from build123d import *

# Parameters (mm, degrees)
SKETCH1_W           = 16
SKETCH1_H           = 25
SKETCH1_W_2         = 11
SKETCH1_H_2         = 20
BOSS_EXTRUDE2_DEPTH = 2.5
SKETCH1_4_W         = 2.5
SKETCH1_4_H         = 2.5
BOSS_EXTRUDE3_DEPTH = 40
BOSS_EXTRUDE4_START = 40
SKETCH1_5_W         = 2.5
SKETCH1_5_H         = 20
SKETCH1_5_H_2       = 2.5
SKETCH1_5_W_2       = 11
BOSS_EXTRUDE4_DEPTH = 2.5


with BuildPart() as part:
    # Sketch1 → Boss-Extrude2 (new body)
    with BuildSketch(Plane(origin=(0, 0, 0), x_dir=(1, 0, 0), z_dir=(0, 1, 0))):
        with Locations((-8, 12.5)):
            Rectangle(SKETCH1_W, SKETCH1_H)
        with Locations((-8, 12.5)):
            Rectangle(SKETCH1_W_2, SKETCH1_H_2, mode=Mode.SUBTRACT)
    extrude(amount=BOSS_EXTRUDE2_DEPTH)

    # Sketch1_4 → Boss-Extrude3 (add)
    with BuildSketch(Plane(origin=(0, 0, 0), x_dir=(1, 0, 0), z_dir=(0, 1, 0))):
        with Locations((-14.75, 23.75)):
            Rectangle(SKETCH1_4_W, SKETCH1_4_H)
        with Locations((-14.75, 1.25)):
            Rectangle(SKETCH1_4_W, SKETCH1_4_H)
        with Locations((-1.25, 1.25)):
            Rectangle(SKETCH1_4_W, SKETCH1_4_H)
        with Locations((-1.25, 23.75)):
            Rectangle(SKETCH1_4_W, SKETCH1_4_H)
    extrude(amount=BOSS_EXTRUDE3_DEPTH)

    # Sketch1_5 → Boss-Extrude4 (add)
    with BuildSketch(Plane(origin=(0, 0, 0), x_dir=(1, 0, 0), z_dir=(0, 1, 0)).offset(BOSS_EXTRUDE4_START)):
        with Locations((-1.25, 12.5)):
            Rectangle(SKETCH1_5_W, SKETCH1_5_H)
        with Locations((-1.25, 1.25)):
            Rectangle(SKETCH1_5_W, SKETCH1_5_H_2)
        with Locations((-8, 1.25)):
            Rectangle(SKETCH1_5_W_2, SKETCH1_5_H_2)
        with Locations((-14.75, 1.25)):
            Rectangle(SKETCH1_5_W, SKETCH1_5_H_2)
        with Locations((-14.75, 12.5)):
            Rectangle(SKETCH1_5_W, SKETCH1_5_H)
        with Locations((-14.75, 23.75)):
            Rectangle(SKETCH1_5_W, SKETCH1_5_H_2)
        with Locations((-8, 23.75)):
            Rectangle(SKETCH1_5_W_2, SKETCH1_5_H_2)
        with Locations((-1.25, 23.75)):
            Rectangle(SKETCH1_5_W, SKETCH1_5_H_2)
    extrude(amount=BOSS_EXTRUDE4_DEPTH)


solid = part.part
Work out the finished part from the listing and answer in its coordinate system (mm). A direction names the side the tool comes from. Round coordinates to 2 decimals unless told otherwise and drop trailing zeros. Write each loop counter-clockwise with the first axis right and the second up, starting at its lowest first coordinate (ties: lowest second). Pieces come first, ordered by that corner, then holes. Notation, with made-up numbers: (48.25, 56) - (86.25, 56) arc R37 cw to (86.25, 92) - close; hole circle Ø9 at (47.25, 89.5). An arc over 180 degrees is marked (long way). Answer in a Markdown table with one row per item. Add a question column.
1. A cutting plane is placed at A-A, the plane y = 18. Determine the outline of the cut face in (x, z), and give its area (3 significant figures).
2. A cutting plane is placed at B-B, the plane z = -12.5. Determine the outline of the cut face in (x, y), and give its area (3 significant figures).
3. A cutting plane is placed at D-D, the plane x = -0.75. Determine the outline of the cut face in (y, z), and give its area (4 significant figures).
4. A cutting plane is placed at C-C, the plane z = -23. Determine the outline of the cut face in (x, y).
5. Find the intervals of material crossed by line 1 along Y through (x, z) = (-5.75, -23); line 2 along X through (y, z) = (11, -0.75); line 3 along Z through (x, y) = (-14.5, 38.5), in increasing order. Write a range as from..to.
6. The mould has two halves that part along X. Classify faces 4 (the flat face through (-1, 0, -13)), 5 (the flat face through (-16, 23, -23)), 6 (the flat face through (-13.5, 1, -12)): +X half, -X half, draft (parallel to the pull), parting line (faces both ways), or undercut.
7. For faces 1 (the flat face through (-1, 21, -22.5)), 2 (the flat face through (-13.5, 21, -1)), 3 (the flat face through (-8, 41, -2.5)), determine the directions among +Z, -Z, +X, -X, +Y, -Y from which every point of the face is accessible in a straight line to the end or side of a thin tool.
Worked out:
| question | item | result |
|---|---|---|
| 1 | outline | (-16, -25) - (-13.5, -25) - (-13.5, -22.5) - (-16, -22.5) - close; (-16, -2.5) - (-13.5, -2.5) - (-13.5, 0) - (-16, 0) - close; (-2.5, -25) - (0, -25) - (0, -22.5) - (-2.5, -22.5) - close; (-2.5, -2.5) - (0, -2.5) - (0, 0) - (-2.5, 0) - close |
| 1 | area | 25.0 mm^2 |
| 2 | outline | (-16, 0) - (-13.5, 0) - (-13.5, 2.5) - (-16, 2.5) - close; (-16, 40) - (-13.5, 40) - (-13.5, 42.5) - (-16, 42.5) - close; (-2.5, 0) - (0, 0) - (0, 2.5) - (-2.5, 2.5) - close; (-2.5, 40) - (0, 40) - (0, 42.5) - (-2.5, 42.5) - close |
| 2 | area | 25.0 mm^2 |
| 3 | outline | (0, -25) - (42.5, -25) - (42.5, 0) - (0, 0) - close; hole (2.5, -22.5) - (40, -22.5) - (40, -2.5) - (2.5, -2.5) - close |
| 3 | area | 312.5 mm^2 |
| 4 | outline | (-16, 0) - (0, 0) - (0, 42.5) - (-16, 42.5) - close; hole (-13.5, 2.5) - (-2.5, 2.5) - (-2.5, 40) - (-13.5, 40) - close |
| 5 | line 1 | 0..2.5, 40..42.5 |
| 5 | line 2 | -16..-13.5, -2.5..0 |
| 5 | line 3 | -25..-22.5, -2.5..0 |
| 6 | face 4 | draft |
| 6 | face 5 | -X half |
| 6 | face 6 | undercut |
| 7 | face 1 | +X, -X |
| 7 | face 2 | +Z, -Z |
| 7 | face 3 | +Y, -Y |
